from build123d import *

# Parameters (mm, degrees)
BOSS_EXTRUDE5_DEPTH = 0.5
BOSS_EXTRUDE6_DEPTH = 0.5
BOSS_EXTRUDE7_DEPTH = 0.5


with BuildPart() as part:
    # Sketch2 → Boss-Extrude5 (new body)
    with BuildSketch(Plane(origin=(0, 0, 0), x_dir=(1, 0, 0), z_dir=(0, 1, 0))):
        Polygon((0, 10), (0, 0), (10, 0), align=None)
    extrude(amount=BOSS_EXTRUDE5_DEPTH)

    # Sketch3 → Boss-Extrude6 (add)
    with BuildSketch(Plane.XY):
        Polygon((0, 0), (0, 10), (10, 0), align=None)
    extrude(amount=-BOSS_EXTRUDE6_DEPTH)

    # Sketch4 → Boss-Extrude7 (add)
    with BuildSketch(Plane.ZY):
        Polygon((-10, 0), (0, 0), (0, 10), align=None)
    extrude(amount=-BOSS_EXTRUDE7_DEPTH)


solid = part.part
Build history of the part. All positions in model axes, mm. A direction names the side the tool comes from. Round coordinates to 2 decimals unless told otherwise and drop trailing zeros. Loops run counter-clockwise (first coordinate to the right, second up) from the corner with the lowest first, then second, coordinate; pieces in that order, holes last. Notation, with made-up numbers: (-10.5, -20.5) -> (4.5, -20.5) arc R8 cw to (4.5, -11.5) -> close; hole circle Ø7 at (-23, 58.25). An arc over 180 degrees is marked (long way). One line per item, written item: value. Start each with the question number.
Q1. Cut at B-B on z = -1.75. List the corners of the cut face in (x, y).
Q2. Probe line 1 along Y through (x, z) = (0.75, -8.75); line 2 along Z through (x, y) = (2.75, 1.5). List the from-to ranges inside material, lowest first.
Q3. Cut at A-A on y = 5.75. List the corners of the cut face in (x, z), plus the area to 3 significant figures.
Q4. Drop flat-ended pins along their axis: pin 1 Ø4.5 at (x, y) = (4.5, 4) entering from -Z; pin 2 Ø1 at (x, y) = (4.5, 6.5) entering from +Z. Give the stop position or say it passes through.
Q5. 3-axis set-ups, long thin cutter, end or side, ignore diameter. For faces 1 (the face through (5.1, 0.2, -4.9)), 2 (the face through (3, 3, -0.5)): which of +Z, -Z, +X, -X, +Y, -Y reach the whole face in a straight line?
Computed:
1. outline: (0, 0) -> (8.25, 0) -> (8.25, 0.5) -> (0.5, 0.5) -> (0.5, 8.25) -> (0, 8.25) -> close
2. line 1: 0 to 0.5
2. line 2: -0.5 to 0
3. outline: (0, -4.25) -> (0.5, -4.25) -> (0.5, -0.5) -> (4.25, -0.5) -> (4.25, 0) -> (0, 0) -> close
3. area: 4.00 mm²
4. pin 1: z = -0.5
4. pin 2: through
5. face 1: -Z, +X, +Y, -Y
5. face 2: -Z, +X, +Y
